Check sheet for the modelled part. Datum: model origin and axes. Units: mm. Face numbers are marked on the shaded views. A direction names the side the tool comes from. Round coordinates to 2 decimals unless told otherwise and drop trailing zeros. Write each loop counter-clockwise with the first axis right and the second up, starting at its lowest first coordinate (ties: lowest second). Pieces come first, ordered by that corner, then holes. Notation, with made-up numbers: (-7, 29.5) -> (-2, 29.5) arc R23 cw to (-2, 60.5) -> close; hole circle Ø4 at (61, 82). An arc over 180 degrees is marked (long way). Answer as a JSON object with one key per item and string values. Group by question number.
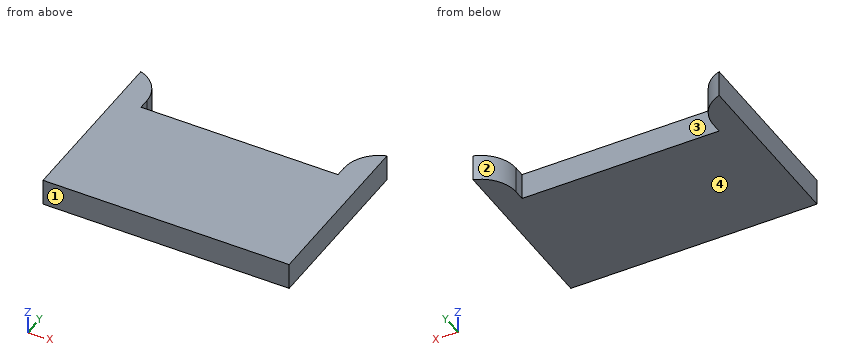
```python
from build123d import *

# Parameters (mm, degrees)
BOSS_EXTRUDE1_DEPTH = 6
FILLET7_R           = 8
FILLET8_R           = 8


with BuildPart() as part:
    # Sketch1 → Boss-Extrude1 (new body)
    with BuildSketch(Plane.XY):
        Polygon((-27.927868544, -36.616915423), (27.927868544, -36.616915423), (27.927868544, 3.383084577), (22.35572924, 3.383084577), (22.35572924, -6.616915423), (-22.35572924, -6.616915423), (-22.35572924, 3.383084577), (-27.927868544, 3.383084577), align=None)
    extrude(amount=BOSS_EXTRUDE1_DEPTH)

    # Fillet7
    # the kernel refuses this fillet: 8 mm, written as the material it takes off along each edge
    with BuildSketch(Plane(origin=(-22.35572924, 3.383084577, -19.056739693), x_dir=(0, -1, 0), z_dir=(0, 0, 1))) as fillet7_piece_1:
        with BuildLine():
            CenterArc((7.622695877, -8), FILLET7_R, 90, 72.333104018)
            Line((0, -5.572139303), (-0.152453918, -5.52358209))
            ThreePointArc((-0.152453918, -5.52358209), (-0.16, -2.786069652), (-0.16, 0))
            Line((-0.16, 0), (0, 0.16))
            Line((0, 0.16), (7.622695877, 0.16))
            Line((7.622695877, 0.16), (7.622695877, 0))
        make_face()
    extrude(amount=44.113479387, mode=Mode.SUBTRACT)

    # Fillet8
    # the kernel refuses this fillet: 8 mm, written as the material it takes off along each edge
    with BuildSketch(Plane(origin=(22.35572924, 3.383084577, -19.056739693), x_dir=(1, 0, 0), z_dir=(0, 0, 1))) as fillet8_piece_1:
        with BuildLine():
            CenterArc((8, -7.622695877), FILLET8_R, 107.666895982, 72.333104018)
            Line((0, -7.622695877), (-0.16, -7.622695877))
            Line((-0.16, -7.622695877), (-0.16, 0))
            Line((-0.16, 0), (0, 0.16))
            ThreePointArc((0, 0.16), (2.786069652, 0.16), (5.52358209, 0.152453918))
            Line((5.52358209, 0.152453918), (5.572139303, 0))
        make_face()
    extrude(amount=44.113479387, mode=Mode.SUBTRACT)


solid = part.part
```
(1) Go/stop test with a flat-tipped pin: pin 1 Ø1.8 at (x, z) = (3, 4) entering from +Y. Record where the tip stops, or that it passes through.
(2) Section check A-A on y = -3. Record the cut outline in (x, z), then the cut area to 3 significant figures.
(3) Release check for a two-part mould opening along X. For the marked faces 3 and 4 record: pulls with the +X half, pulls with the -X half, needs draft (parallel to the pull), parting line crosses it, or undercut.
(4) Access from +Z, -Z, +X, -X, +Y, -Y to the whole of each face (thin tool, end or side, straight path). Record for the marked faces 1 and 2.
(5) Section check C-C on x = -4. Record the cut outline in (y, z), then the cut area to 3 significant figures.
(6) Scan lines: line 1 along X through (y, z) = (-5.5, 2.6); line 2 along X through (y, z) = (0.5, 4.4); line 3 along Y through (x, z) = (-21, 3.4). Record each from-to range of solid material in increasing order.
(7) Section check B-B on z = 4.7. Record the cut outline in (x, y), then the cut area to 3 significant figures.
Data:
{
 "1": {"pin 1": "stops at y = -6.62"},
 "2": {"outline": "(-27.93, 0) -> (-22.45, 0) -> (-22.45, 6) -> (-27.93, 6) -> close; (22.45, 0) -> (27.93, 0) -> (27.93, 6) -> (22.45, 6) -> close", "area": "65.7 mm²"},
 "3": {"face 3": "undercut", "face 4": "needs draft"},
 "4": {"face 1": "+Z, -Z, +X, -X, -Y", "face 2": "+Z, -Z, +Y"},
 "5": {"outline": "(-36.62, 0) -> (-6.62, 0) -> (-6.62, 6) -> (-36.62, 6) -> close", "area": "180 mm²"},
 "6": {"line 1": "x = -27.93 to -22.36, 22.36 to 27.93", "line 2": "x = -27.93 to -23.91, 23.91 to 27.93", "line 3": "y = -36.62 to -6.62"},
 "7": {"outline": "(-27.93, -36.62) -> (27.93, -36.62) -> (27.93, 3.38) arc R8 ccw to (22.36, -4.24) -> (22.36, -6.62) -> (-22.36, -6.62) -> (-22.36, -4.24) arc R8 ccw to (-27.93, 3.38) -> close", "area": "1,760 mm²"}
}
